Source: CAD feature listing. Evaluate the final solid. Frame: model axes, mm. A direction names the side the tool comes from. Give positions to 0.01 mm unless a question says otherwise; leave off trailing zeros. Write each loop counter-clockwise with the first axis right and the second up, starting at its lowest first coordinate (ties: lowest second). Pieces come first, ordered by that corner, then holes. Notation, with made-up numbers: (39, 22.5) - (77, 22.5) arc R11 ccw to (77, 40.5) - close; hole circle Ø9 at (78, 84.25). An arc over 180 degrees is marked (long way). Answer as a JSON object with one key per item and string values. Group by question number.
from build123d import *

# Parameters (mm, degrees)
F0_W     = 635
F0_H     = 2500
F1_DEPTH = 18
F2_W     = 635
F2_H     = 1648
F3_DEPTH = 6


with BuildPart() as f1:
    # F0 (on Right) → F1 (new body)
    with BuildSketch(Plane.YZ):
        Rectangle(F0_W, F0_H)
    extrude(amount=F1_DEPTH)

    # F2 (on face) → F3 (cut)
    with BuildSketch(Plane(origin=(0, 0, 0), x_dir=(0, -1, 0), z_dir=(-1, 0, 0))):
        with Locations((0, 426)):
            Rectangle(F2_W, F2_H)
    extrude(amount=-F3_DEPTH, mode=Mode.SUBTRACT)


solid = f1.part
Q1. Section A-A on y = 261. Return the cut outline in (x, z), then the cut area to 3 significant figures.
Q2. Ray query, probe 1 along X at (y, z) = (-145.5, 991); probe 2 along Z at (x, y) = (4.25, -192). Return the intervals inside material, ascending. Write a range as [from, to].
Q3. First-contact query: pin 1 Ø8 at (y, z) = (-137, 2) entering from -X; pin 2 Ø1.8 at (x, y) = (1.5, -84) entering from +Z. Flat tips, straight axial feed; report the tip coordinate or a pass-through.
Q4. Section B-B on z = 4. Return the cut outline in (x, y), then the cut area to 3 significant figures.
Q5. Reachability of faces 1 (the flat face through (0, -4, -818)), 2 (the flat face through (6, 4, 438)) from +Z, -Z, +X, -X, +Y, -Y: full face, straight path, thin tool, end or side. Return the list, or none.
Taken from the geometry:
{
 "1": {"outline": "(0, -1250) - (18, -1250) - (18, 1250) - (6, 1250) - (6, -398) - (0, -398) - close", "area": "35,100 mm²"},
 "2": {"probe 1": "x = [6, 18]", "probe 2": "z = [-1250, -398]"},
 "3": {"pin 1": "stops at x = 6", "pin 2": "stops at z = -398"},
 "4": {"outline": "(6, -317.5) - (18, -317.5) - (18, 317.5) - (6, 317.5) - close", "area": "7,620 mm²"},
 "5": {"face 1": "+Z, -Z, -X, +Y, -Y", "face 2": "+Z, -X, +Y, -Y"}
}
